```python
from build123d import *

# Parameters (mm, degrees)
SKETCH1_R           = 3.429
SKETCH1_R_2         = 2.54
BOSS_EXTRUDE1_DEPTH = 3.2004
SKETCH2_R           = 2.413
CUT_EXTRUDE1_DEPTH  = 3.2004
SKETCH3_R           = 2.159
CUT_EXTRUDE2_DEPTH  = 3.2004
SKETCH6_W           = 107.95
SKETCH6_H           = 3.2512
CUT_EXTRUDE3_DEPTH  = 3.2004
SKETCH7_R           = 3.429
CUT_EXTRUDE4_DEPTH  = 3.2004
CUT_EXTRUDE5_START  = -3.2004
CUT_EXTRUDE5_DEPTH  = 3.2004
CUT_EXTRUDE6_START  = -3.2004
CUT_EXTRUDE6_DEPTH  = 3.2004
BOSS_EXTRUDE2_DEPTH = 3.2004
SKETCH13_R          = 1.1303
CUT_EXTRUDE7_DEPTH  = 3.2004
CUT_EXTRUDE8_DEPTH  = 3.2004
FILLET1_R           = 5.08
SKETCH16_R          = 1.1303
CUT_EXTRUDE9_DEPTH  = 3.2004
SKETCH20_R          = 2.159
CUT_EXTRUDE11_DEPTH = 3.2004
CUT_EXTRUDE12_DEPTH = 3.2004
FILLET2_R           = 5.08


with BuildPart() as part:
    # Sketch1 → Boss-Extrude1 (new body)
    with BuildSketch(Plane.XY):
        with BuildLine():
            Line((0, 0), (120.015, 0))
            ThreePointArc((120.015, 0), (130.351788396, 3.075697789), (137.325636158, 11.302152592))
            Line((137.325636158, 11.302152592), (155.2575, 52.11572))
            ThreePointArc((155.2575, 52.11572), (157.54731739, 67.602183396), (151.630955452, 82.09599151))
            ThreePointArc((151.630955452, 82.09599151), (60.0075, 127.266502568), (-31.615955452, 82.09599151))
            ThreePointArc((-31.615955452, 82.09599151), (-37.53231739, 67.602183396), (-35.2425, 52.11572))
            Line((-35.2425, 52.11572), (-17.310636158, 11.302152592))
            ThreePointArc((-17.310636158, 11.302152592), (-10.336788396, 3.075697789), (0, 0))
        make_face()
        with Locations((120.015, 18.90776)):
            Circle(SKETCH1_R, mode=Mode.SUBTRACT)
        with Locations((0, 18.90776)):
            Circle(SKETCH1_R_2, mode=Mode.SUBTRACT)
        with Locations((19.734727626, 25.566426992)):
            Circle(SKETCH1_R_2, mode=Mode.SUBTRACT)
    extrude(amount=BOSS_EXTRUDE1_DEPTH)

    # Sketch2 → Cut-Extrude1 (cut)
    with BuildSketch(Plane(origin=(0, 0, 0), x_dir=(-1, 0, 0), z_dir=(0, 0, -1))):
        with Locations((-92.0115, 52.11572)):
            Circle(SKETCH2_R)
        with Locations((-76.0095, 52.11572)):
            Circle(SKETCH2_R)
        with Locations((-44.0055, 52.11572)):
            Circle(SKETCH2_R)
        with Locations((-28.0035, 52.11572)):
            Circle(SKETCH2_R)
    extrude(amount=-CUT_EXTRUDE1_DEPTH, mode=Mode.SUBTRACT)

    # Sketch3 → Cut-Extrude2 (cut)
    with BuildSketch(Plane.XY.offset(3.2004)):
        with Locations((21.9075, 3.81)):
            Circle(SKETCH3_R)
        with Locations((60.0075, 3.81)):
            Circle(SKETCH3_R)
        with Locations((98.1075, 3.81)):
            Circle(SKETCH3_R)
    extrude(amount=-CUT_EXTRUDE2_DEPTH, mode=Mode.SUBTRACT)

    # Sketch6 → Cut-Extrude3 (cut)
    with BuildSketch(Plane(origin=(0, 0, 0), x_dir=(-1, 0, 0), z_dir=(0, 0, -1))):
        with Locations((-60.0075, 46.68012)):
            Rectangle(SKETCH6_W, SKETCH6_H)
    extrude(amount=-CUT_EXTRUDE3_DEPTH, mode=Mode.SUBTRACT)

    # Sketch7 → Cut-Extrude4 (cut)
    with BuildSketch(Plane.XY.offset(3.2004)):
        with Locations((126.474462556, 80.535782848)):
            Circle(SKETCH7_R)
    extrude(amount=-CUT_EXTRUDE4_DEPTH, mode=Mode.SUBTRACT)

    # Sketch11 → Cut-Extrude5 (cut)
    with BuildSketch(Plane.XY.offset(3.2004).offset(CUT_EXTRUDE5_START)):
        with BuildLine():
            Line((121.158447362, 109.75190519), (95.966712331, 89.752651283))
            Line((95.966712331, 89.752651283), (35.832210764, 94.542990135))
            Line((35.832210764, 94.542990135), (38.27464621, 125.20358486))
            ThreePointArc((38.27464621, 125.20358486), (81.176702308, 125.310112932), (121.158447362, 109.75190519))
        make_face()
    extrude(amount=CUT_EXTRUDE5_DEPTH, mode=Mode.SUBTRACT)

    # Sketch12 → Cut-Extrude6 (cut)
    with BuildSketch(Plane.XY.offset(3.2004).offset(CUT_EXTRUDE6_START)):
        with BuildLine():
            Line((36.857132229, 114.618997738), (37.427852032, 114.573533967))
            Line((37.427852032, 114.573533967), (38.27464621, 125.20358486))
            ThreePointArc((38.27464621, 125.20358486), (31.851547204, 123.782382999), (25.51977184, 121.997828065))
            ThreePointArc((25.51977184, 121.997828065), (30.251350905, 116.868583991), (36.857132229, 114.618997738))
        make_face()
    extrude(amount=CUT_EXTRUDE6_DEPTH, mode=Mode.SUBTRACT)

    # Sketch14 → Boss-Extrude2 (add)
    with BuildSketch(Plane.XY.offset(3.2004)):
        with BuildLine():
            Line((-45.169534314, 54.57440881), (-19.78010381, 11.324779025))
            ThreePointArc((-19.78010381, 11.324779025), (-11.396305615, 3.031534227), (0, 0))
            ThreePointArc((0, 0), (-12.750544623, 66.33524155), (25.51977184, 121.997828065))
            ThreePointArc((25.51977184, 121.997828065), (-11.283339646, 106.926625279), (-42.217820701, 81.933265153))
            ThreePointArc((-42.217820701, 81.933265153), (-48.214081814, 68.741537884), (-45.169534314, 54.57440881))
        make_face()
    extrude(amount=-BOSS_EXTRUDE2_DEPTH)

    # Sketch13 → Cut-Extrude7 (cut)
    with BuildSketch(Plane.XY.offset(3.2004)):
        with Locations((50.4825, 81.07172)):
            Circle(SKETCH13_R)
        with Locations((50.4825, 60.75172)):
            Circle(SKETCH13_R)
        with Locations((25.0825, 60.75172)):
            Circle(SKETCH13_R)
        with Locations((25.0825, 81.07172)):
            Circle(SKETCH13_R)
        with Locations((12.3825, 81.07172)):
            Circle(SKETCH13_R)
        with Locations((12.3825, 60.75172)):
            Circle(SKETCH13_R)
        with Locations((-13.0175, 60.75172)):
            Circle(SKETCH13_R)
        with Locations((-13.0175, 81.07172)):
            Circle(SKETCH13_R)
    extrude(amount=-CUT_EXTRUDE7_DEPTH, mode=Mode.SUBTRACT)

    # Sketch15 → Cut-Extrude8 (cut)
    with BuildSketch(Plane.XY.offset(3.2004)):
        with BuildLine():
            Line((79.0575, 73.70572), (104.4575, 73.70572))
            ThreePointArc((104.4575, 73.70572), (110.8075, 67.35572), (104.4575, 61.00572))
            Line((104.4575, 61.00572), (79.0575, 61.00572))
            ThreePointArc((79.0575, 61.00572), (72.7075, 67.35572), (79.0575, 73.70572))
        make_face()
        with BuildLine():
            Line((78.4225, 22.08276), (97.4725, 22.08276))
            ThreePointArc((97.4725, 22.08276), (100.6475, 18.90776), (97.4725, 15.73276))
            Line((97.4725, 15.73276), (78.4225, 15.73276))
            ThreePointArc((78.4225, 15.73276), (75.2475, 18.90776), (78.4225, 22.08276))
        make_face()
    extrude(amount=-CUT_EXTRUDE8_DEPTH, mode=Mode.SUBTRACT)

    # Fillet1
    fillet1_edges = [part.edges().sort_by_distance(p)[0] for p in [
        (121.158447362, 109.75190519, 1.6002),
        (37.427852032, 114.573533967, 1.6002),
        (25.51977184, 121.997828065, 1.6002),
    ]]
    fillet(fillet1_edges, radius=FILLET1_R)

    # Sketch16 → Cut-Extrude9 (cut)
    with BuildSketch(Plane.XY.offset(3.2004)):
        with Locations((112.438115095, 24.679799513)):
            Circle(SKETCH16_R)
        with Locations((127.591884905, 13.135720487)):
            Circle(SKETCH16_R)
    extrude(amount=-CUT_EXTRUDE9_DEPTH, mode=Mode.SUBTRACT)

    # Sketch20 → Cut-Extrude11 (cut)
    with BuildSketch(Plane.XY.offset(3.2004)):
        with Locations((8.255, 18.90776)):
            Circle(SKETCH20_R)
        with Locations((107.05592, 18.90776)):
            Circle(SKETCH20_R)
    extrude(amount=-CUT_EXTRUDE11_DEPTH, mode=Mode.SUBTRACT)

    # Sketch21 → Cut-Extrude12 (cut)
    with BuildSketch(Plane(origin=(0, 0, 0), x_dir=(-1, 0, 0), z_dir=(0, 0, -1))):
        Polygon((16.731556446, 111.864036412), (21.254933404, 60.933416848), (65.105179276, 65.815561516), align=None)
    extrude(amount=-CUT_EXTRUDE12_DEPTH, mode=Mode.SUBTRACT)

    # Fillet2
    fillet2_edges = [part.edges().sort_by_distance(p)[0] for p in [
        (-48.229671102, 63.936696971, 1.6002),
        (-17.517967545, 103.009500331, 1.6002),
        (-21.254933404, 60.933416848, 1.6002),
    ]]
    fillet(fillet2_edges, radius=FILLET2_R)


solid = part.part
```
Build history of the part. All positions in model axes, mm. A direction names the side the tool comes from. Give positions to 0.01 mm unless a question says otherwise; leave off trailing zeros. Order: outer loops, then holes, each group sorted by start corner. A loop starts at its lowest first (then second) coordinate and runs counter-clockwise, first axis right, second up. Notation, with made-up numbers: M 64,33.5 L 79,33.5 A13 cw 79,45.5 Z; hole C 29.5,-17 d3. An arc over 180 degrees is marked long. Return JSON: item names as keys, results as strings.
Q1. Band-saw the part on C-C (z = 0.95). Count the separate pieces of the cut face and the enclosed holes in it, then the cut area to 3 significant figures.
Answer list:
{"separate pieces": "1", "enclosed holes": "26", "area": "16,500 mm^2"}
Q2. Flat gauge pins, fed straight in: pin 1 (1.6 mm diameter, centred on y = 47, z = 1, fed in from +X); pin 2 (1 mm diameter, centred on x = -1.5, z = 1, fed in from +Y). Where does each tip first touch, or does it go through?
Answer list:
{"pin 1": "stops at x = 153.36", "pin 2": "stops at y = 112.43"}
Q3. Two-plate mould, pull along Y, no slides. Class faces 3 (the face through (139.199, 95.848, 1.578)), 4 (the face through (-11.541, 3.115, 1.623)), 5 (the face through (117.49, 21.23, 1.58)), 6 (the face through (110.806, 67.495, 1.623)): pulls with the +Y half, pulls with the -Y half, needs draft (parallel to the pull), parting line crosses it, or undercut.
Answer list:
{"face 3": "pulls with the +Y half", "face 4": "pulls with the -Y half", "face 5": "undercut", "face 6": "undercut"}
Q4. Band-saw the part on B-B (x = 8). Give the cut face in (y, z), then the cut area to 3 significant figures.
Answer list:
{"outline": "M 0,0 L 16.76,0 L 16.76,3.2 L 0,3.2 Z; M 21.05,0 L 45.05,0 L 45.05,3.2 L 21.05,3.2 Z; M 48.31,0 L 116.38,0 L 116.38,3.2 L 48.31,3.2 Z", "area": "348 mm^2"}
Q5. 3-axis set-ups, long thin cutter, end or side, ignore diameter. For faces 1 (the face through (107.29, 98.74, 1.58)), 2 (the face through (123.753, 78.449, 1.623)): which of +Z, -Z, +X, -X, +Y, -Y reach the whole face in a straight line?
Answer list:
{"face 1": "+Z, -Z, +Y", "face 2": "+Z, -Z"}
Q6. Band-saw the part on A-A (y = 3.81). Give the cut face in (x, z).
Answer list:
{"outline": "M -12.66,0 L 19.75,0 L 19.75,3.2 L -12.66,3.2 Z; M 24.07,0 L 57.85,0 L 57.85,3.2 L 24.07,3.2 Z; M 62.17,0 L 95.95,0 L 95.95,3.2 L 62.17,3.2 Z; M 100.27,0 L 131.4,0 L 131.4,3.2 L 100.27,3.2 Z"}
Q7. Wall check: probe 1 along Y at (x, z) = (108.5, 1.45); probe 2 along Y at (x, z) = (26.5, 2.8); probe 3 along X at (y, z) = (21.5, 2.85). Give the ranges that are in metal, low to high. Write a range as from..to.
Answer list:
{"probe 1": "y = 0..17.3, 20.51..45.05, 48.31..62.46, 72.25..99.7", "probe 2": "y = 0..45.05, 48.31..50.23, 54..120.2", "probe 3": "x = -25.75..76.59, 99.31..117.77, 122.26..141.81"}
